The figure shows three views and two pictorial views of one solid part (mm, origin at its lowest corner). Answer the questions. A direction names the side the tool comes from. Give positions to 0.01 mm unless a question says otherwise; leave off trailing zeros. Order: outer loops, then holes, each group sorted by start corner. A loop starts at its lowest first (then second) coordinate and runs counter-clockwise, first axis right, second up. Notation, with made-up numbers: (76, 12.5) - (109, 12.5) arc R15 ccw to (109, 25.5) - close; hole circle Ø5 at (-35.5, -32.5). An arc over 180 degrees is marked (long way). Use a Markdown table: item, result. Add a question column.
1. For a pull along Z with two mould halves and no side action, classify the marked faces 4, 5 and 6 as released by +Z, released by -Z, zero draft, split by the parting line, or undercut.
2. Consider L1, parallel to X at y = 4.2, z = 17.25; L2, parallel to X at y = 1.05, z = 17.1; L3, parallel to Z at x = 35, y = 1.5. Determine where each line is inside the solid, lowest interval first.
3. A cutting plane is placed at D-D on y = 1.1. Determine the outline of the cut face in (x, z), and give its area (3 significant figures).
4. A cutting plane is placed at B-B on z = 3. Determine the outline of the cut face in (x, y), and give its area (3 significant figures).
5. A cutting plane is placed at C-C on x = 33.5. Determine the outline of the cut face in (y, z).
6. Flat-ended cylindrical pins translate along their axes: P1, Ø3, axis at x = 34.6, z = 3, coming from the +Y side; P2, Ø12, axis at x = 8.5, z = 7, coming from the +Y side; P3, Ø2, axis at y = 1, z = 8.5, coming from the -X side; P4, Ø4, axis at x = 23, z = 13.5, coming from the +Y side. Find the tip coordinate at first contact, or state that the pin passes through.
7. A cutting plane is placed at A-A on y = 3. Determine the outline of the cut face in (x, z).
8. Which of the six approach directions +Z, -Z, +X, -X, +Y, -Y give full straight-line access (tool end or side, diameter ignored) to the marked faces 1, 2 and 3?
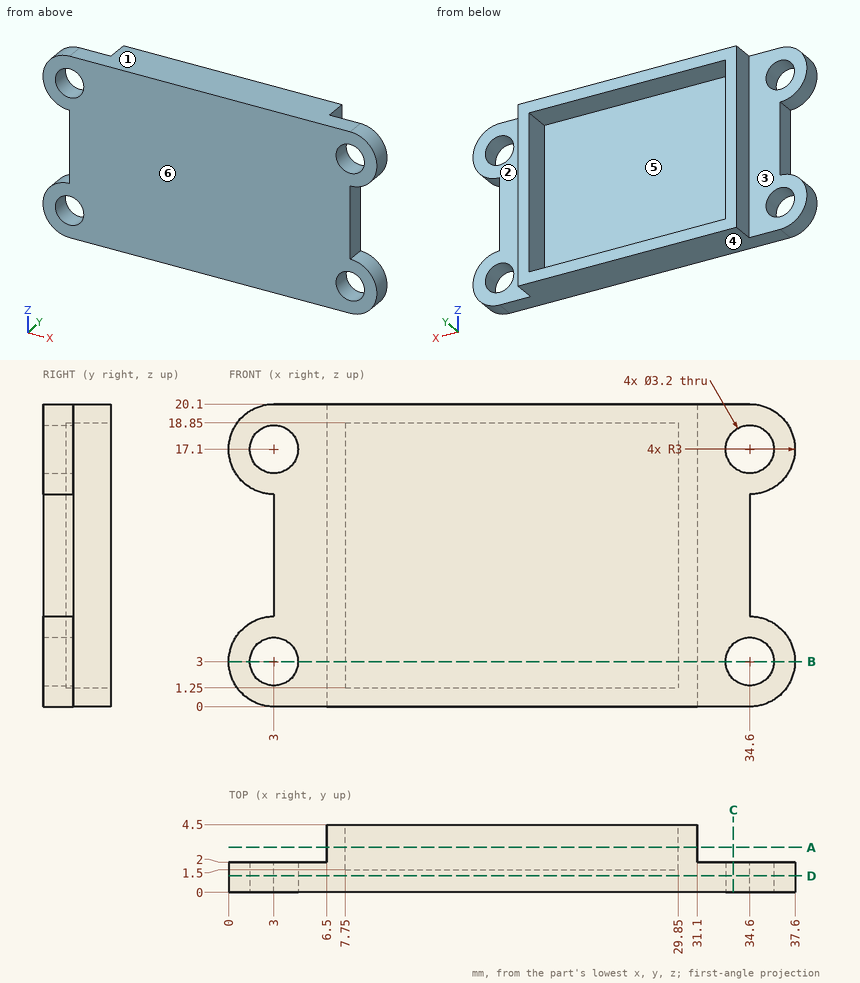
Output values:
| question | item | result |
|---|---|---|
| 1 | face 4 | released by -Z |
| 1 | face 5 | undercut |
| 1 | face 6 | zero draft |
| 2 | L1 | 6.5 to 7.75, 29.85 to 31.1 |
| 2 | L2 | 0 to 1.4, 4.6 to 33, 36.2 to 37.6 |
| 2 | L3 | 0.03 to 1.45, 4.55 to 5.97, 14.13 to 15.55, 18.65 to 20.07 |
| 3 | outline | (3, 0) - (34.6, 0) arc R3 ccw to (34.6, 6) - (34.6, 14.1) arc R3 ccw to (34.6, 20.1) - (3, 20.1) arc R3 ccw to (3, 14.1) - (3, 6) arc R3 ccw to start; hole circle Ø3.2 at (3, 3); hole circle Ø3.2 at (3, 17.1); hole circle Ø3.2 at (34.6, 3); hole circle Ø3.2 at (34.6, 17.1) |
| 3 | area | 660 mm² |
| 4 | outline | (0, 0) - (1.4, 0) - (1.4, 2) - (0, 2) - close; (4.6, 0) - (33, 0) - (33, 2) - (31.1, 2) - (31.1, 4.5) - (29.85, 4.5) - (29.85, 1.5) - (7.75, 1.5) - (7.75, 4.5) - (6.5, 4.5) - (6.5, 2) - (4.6, 2) - close; (36.2, 0) - (37.6, 0) - (37.6, 2) - (36.2, 2) - close |
| 4 | area | 57.6 mm² |
| 5 | outline | (0, 0) - (2, 0) - (2, 1.84) - (0, 1.84) - close; (0, 4.16) - (2, 4.16) - (2, 15.94) - (0, 15.94) - close; (0, 18.26) - (2, 18.26) - (2, 20.1) - (0, 20.1) - close |
| 6 | P1 | through |
| 6 | P2 | y = 4.5 |
| 6 | P3 | x = 3 |
| 6 | P4 | y = 1.5 |
| 7 | outline | (6.5, 0) - (31.1, 0) - (31.1, 20.1) - (6.5, 20.1) - close; hole (7.75, 1.25) - (29.85, 1.25) - (29.85, 18.85) - (7.75, 18.85) - close |
| 8 | face 1 | +Z, +X, -X, +Y, -Y |
| 8 | face 2 | +Z, -Z, +X, +Y |
| 8 | face 3 | +Z, -Z, -X, +Y |
